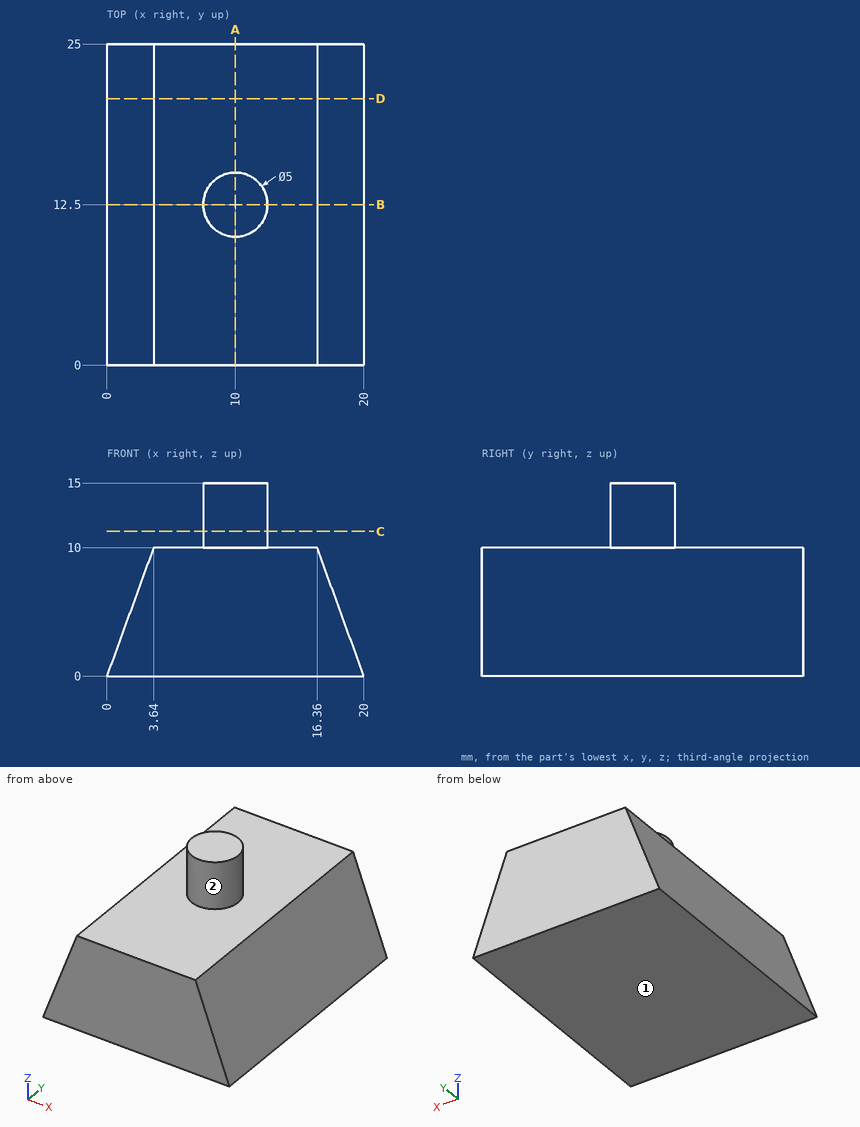
Check sheet for the drawn part. Datum: minimum x, y, z corner. Units: mm. A direction names the side the tool comes from. Round coordinates to 2 decimals unless told otherwise and drop trailing zeros. Loops run counter-clockwise (first coordinate to the right, second up) from the corner with the lowest first, then second, coordinate; pieces in that order, holes last. Notation, with made-up numbers: (61, 30.25) - (77, 30.25) arc R33 cw to (77, 61.25) - close; hole circle Ø7 at (-8.75, 14.25). An arc over 180 degrees is marked (long way). Write each question's results on one line, items separated by ' | '. Start each with the question number.
Q1. Cross-section at C-C on z = 11.25. Enter the section's corners in (x, y), and give its area (3 significant figures).
Q2. Gauge pin test, flat ends, axial feed: P1, Ø1, axis at y = 10.5, z = 5, coming from the +X side; P2, Ø4, axis at x = 11, y = 10, coming from the +Z side. Record the tip position at first contact, or that the pin passes through.
Q3. Thickness scan on line 1 (Z direction, x = 15.75, y = 7.5); line 2 (X direction, y = 5.5, z = 9.75); line 3 (X direction, y = 15.25, z = 2.25). Record the ranges inside material, lowest first. Write a range as [from, to].
Q4. Cross-section at D-D on y = 20.75. Enter the section's corners in (x, z).
Q5. Access from +Z, -Z, +X, -X, +Y, -Y to the whole of each face (thin tool, end or side, straight path). Record for the marked faces 1 and 2.
Q6. Cross-section at A-A on x = 10. Enter the section's corners in (y, z), and give its area (3 significant figures).
Q7. Cross-section at B-B on y = 12.5. Enter the section's corners in (x, z), and give its area (3 significant figures).
Answers below:
1) outline: circle Ø5 at (10, 12.5) | area: 19.6 mm²
2) P1: stops at x = 18.36 | P2: stops at z = 15
3) line 1: z = [0, 10] | line 2: x = [3.55, 16.45] | line 3: x = [0.82, 19.18]
4) outline: (0, 0) - (20, 0) - (16.36, 10) - (3.64, 10) - close
5) face 1: -Z, +X, -X, +Y, -Y | face 2: +Z
6) outline: (0, 0) - (25, 0) - (25, 10) - (15, 10) - (15, 15) - (10, 15) - (10, 10) - (0, 10) - close | area: 275 mm²
7) outline: (0, 0) - (20, 0) - (16.36, 10) - (12.5, 10) - (12.5, 15) - (7.5, 15) - (7.5, 10) - (3.64, 10) - close | area: 189 mm²
